```python
from build123d import *

# Parameters (mm, degrees)
BOSS_EXTRUDE1_DEPTH = 276.225
SKETCH3_R           = 2.667
CUT_EXTRUDE2_DEPTH  = 3.175
SKETCH4_R           = 3.302
SKETCH4_R_2         = 2.4765
CUT_EXTRUDE3_DEPTH  = 3.175
SKETCH8_R           = 2.4765
CUT_EXTRUDE5_DEPTH  = 3.175
SKETCH9_R           = 3.175
CUT_EXTRUDE6_DEPTH  = 3.175


with BuildPart() as part:
    # Sketch1 → Boss-Extrude1 (new body)
    with BuildSketch(Plane.XY):
        with BuildLine():
            Line((3.175, 50.8), (3.175, 3.937))
            ThreePointArc((3.175, 3.937), (3.398184633, 3.398184633), (3.937, 3.175))
            Line((3.937, 3.175), (25.4, 3.175))
            Line((25.4, 3.175), (25.4, 0))
            Line((25.4, 0), (0.762, 0))
            ThreePointArc((0.762, 0), (0.223184633, 0.223184633), (0, 0.762))
            Line((0, 0.762), (0, 50.8))
            Line((0, 50.8), (3.175, 50.8))
        make_face()
    extrude(amount=BOSS_EXTRUDE1_DEPTH)

    # Sketch3 → Cut-Extrude2 (cut)
    with BuildSketch(Plane.XZ):
        with Locations(Location((12.7, 269.875, 0), (0, 0, 270))):
            Circle(SKETCH3_R)
    extrude(amount=-CUT_EXTRUDE2_DEPTH, mode=Mode.SUBTRACT)

    # Sketch4 → Cut-Extrude3 (cut)
    with BuildSketch(Plane(origin=(3.175, 0, 0), x_dir=(0, 0, -1), z_dir=(1, 0, 0))):
        with Locations(Location((-188.9125, 31.75, 0), (0, 0, 90))):
            Circle(SKETCH4_R)
        with Locations(Location((-236.5375, 31.75, 0), (0, 0, 90))):
            Circle(SKETCH4_R)
        with Locations(Location((-133.985, 16.002, 0), (0, 0, 90))):
            Circle(SKETCH4_R_2)
        with Locations(Location((-133.985, 35.052, 0), (0, 0, 90))):
            Circle(SKETCH4_R_2)
    extrude(amount=-CUT_EXTRUDE3_DEPTH, mode=Mode.SUBTRACT)

    # Sketch8 → Cut-Extrude5 (cut)
    with BuildSketch(Plane.ZY):
        with Locations((153.898092, 39.759636)):
            Circle(SKETCH8_R)
    extrude(amount=-CUT_EXTRUDE5_DEPTH, mode=Mode.SUBTRACT)

    # Sketch9 → Cut-Extrude6 (cut)
    with BuildSketch(Plane(origin=(0, 3.175, 0), x_dir=(1, 0, 0), z_dir=(0, 1, 0))):
        with Locations(Location((15.24, -16.686276, 0), (0, 0, 270))):
            Circle(SKETCH9_R)
    extrude(amount=-CUT_EXTRUDE6_DEPTH, mode=Mode.SUBTRACT)


solid = part.part
```
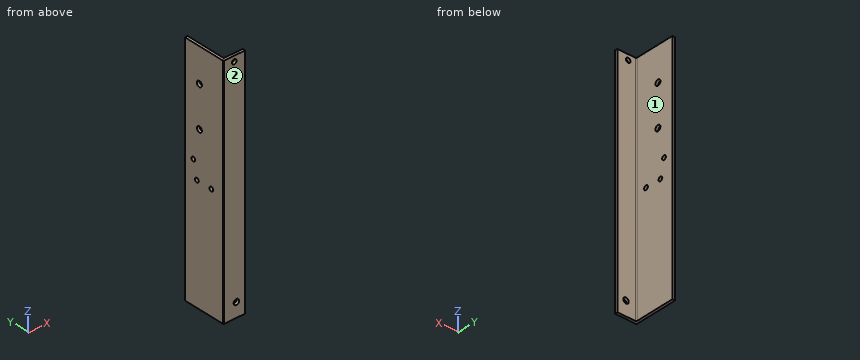
Model file for the job. Use its own axes, mm. Face numbers are marked on the shaded views. A direction names the side the tool comes from. Coordinates: 2 decimals unless noted, no trailing zeros. Write each loop counter-clockwise with the first axis right and the second up, starting at its lowest first coordinate (ties: lowest second). Pieces come first, ordered by that corner, then holes. Notation, with made-up numbers: (-15, 21.25) - (42, 21.25) arc R7 ccw to (42, 31.25) - close; hole circle Ø5 at (-19, 84.5). An arc over 180 degrees is marked (long way). One line per item, written item: value. Start each with the question number.
1. Tool access for the marked faces 1 and 2: list every direction of +Z, -Z, +X, -X, +Y, -Y with a clear straight run to the whole face (end or side of a thin tool).
2. Flat gauge pins, fed straight in: pin 1 (10 mm diameter, centred on x = 12, z = 81, fed in from -Y); pin 2 (4.5 mm diameter, centred on y = 16.002, z = 133.985, fed in from +X); pin 3 (8 mm diameter, centred on y = 15.5, z = 62.5, fed in from +X) (3 decimals); pin 4 (1.5 mm diameter, centred on x = 6, z = 220, fed in from +Y) (3 decimals). Where does each tip first touch, or does it go through?
3. Slice it at A-A (z = 115). Write the cut outline in (x, y) (3 decimals).
4. Probe line 1 (Z direction, x = 1.4, y = 31.75) (1 decimal); line 2 (X direction, y = 41, z = 12.5) (3 decimals). List the from-to ranges inside material, lowest first. Write a range as from..to.
5. Slice it at B-B (y = 8). Write the cut outline in (x, z) (3 decimals).
Answers below:
1. face 1: +Z, -Z, +X, +Y
1. face 2: +Z, -Z, +X, -X, -Y
2. pin 1: stops at y = 0
2. pin 2: passes through
2. pin 3: stops at x = 3.175
2. pin 4: stops at y = 3.175
3. outline: (0, 0.762) arc R0.762 ccw to (0.762, 0) - (25.4, 0) - (25.4, 3.175) - (3.937, 3.175) arc R0.762 cw to (3.175, 3.937) - (3.175, 50.8) - (0, 50.8) - close
4. line 1: z = 0..185.6, 192.2..233.2, 239.8..276.2
4. line 2: x = 0..3.175
5. outline: (0, 0) - (3.175, 0) - (3.175, 276.225) - (0, 276.225) - close
